from build123d import *

# Parameters (mm, degrees)
BOSS_EXTRUDE1_DEPTH = 2.032
FILLET1_R           = 2
SKETCH4_R           = 1.2446
CUT_EXTRUDE1_DEPTH  = 75.115872934
CUT_EXTRUDE2_DEPTH  = 75.115872934


with BuildPart() as part:
    # Sketch3 → Boss-Extrude1 (new body)
    with BuildSketch(Plane.XY):
        with BuildLine():
            Line((62.980794963, 30.66873734), (50.569205037, 30.66873734))
            ThreePointArc((50.569205037, 30.66873734), (45.275, 28.075), (39.980794963, 30.66873734))
            Line((39.980794963, 30.66873734), (27.569205037, 30.66873734))
            ThreePointArc((27.569205037, 30.66873734), (22.275, 28.075), (16.980794963, 30.66873734))
            Line((16.980794963, 30.66873734), (10.658308864, 17.473983742))
            ThreePointArc((10.658308864, 17.473983742), (13.670205209, 16.817167392), (16.069205037, 14.88126266))
            Line((16.069205037, 14.88126266), (28.480794963, 14.88126266))
            ThreePointArc((28.480794963, 14.88126266), (33.775, 17.475), (39.069205037, 14.88126266))
            Line((39.069205037, 14.88126266), (51.480794963, 14.88126266))
            ThreePointArc((51.480794963, 14.88126266), (56.775, 17.475), (62.069205037, 14.88126266))
            Line((62.069205037, 14.88126266), (68.391691136, 28.076016258))
            ThreePointArc((68.391691136, 28.076016258), (65.379794791, 28.732832608), (62.980794963, 30.66873734))
        make_face()
    extrude(amount=BOSS_EXTRUDE1_DEPTH)

    # Fillet1
    fillet1_edges = [part.edges().sort_by_distance(p)[0] for p in [
        (68.391691136, 28.076016258, 1.016),
        (62.069205037, 14.88126266, 1.016),
        (51.480794963, 14.88126266, 1.016),
        (39.069205037, 14.88126266, 1.016),
        (28.480794963, 14.88126266, 1.016),
        (16.069205037, 14.88126266, 1.016),
        (10.658308864, 17.473983742, 1.016),
        (16.980794963, 30.66873734, 1.016),
        (27.569205037, 30.66873734, 1.016),
        (39.980794963, 30.66873734, 1.016),
        (50.569205037, 30.66873734, 1.016),
        (62.980794963, 30.66873734, 1.016),
    ]]
    fillet(fillet1_edges, radius=FILLET1_R)

    # Sketch4 → Cut-Extrude1 (cut, through all)
    with BuildSketch(Plane.XY.offset(2.032)):
        with Locations((22.275, 20.49206771)):
            Circle(SKETCH4_R)
        with Locations((56.775, 25.307013878)):
            Circle(SKETCH4_R)
    extrude(amount=-CUT_EXTRUDE1_DEPTH, mode=Mode.SUBTRACT)

    # Sketch6 → Cut-Extrude2 (cut, through all)
    with BuildSketch(Plane.XY.offset(2.032)):
        with BuildLine():
            Line((62.077939702, 30.66873734), (51.472060298, 30.66873734))
            ThreePointArc((51.472060298, 30.66873734), (50.699880618, 30.513659708), (50.047448735, 30.072475883))
            ThreePointArc((50.047448735, 30.072475883), (45.275, 28.075), (40.502551265, 30.072475883))
            ThreePointArc((40.502551265, 30.072475883), (39.850119382, 30.513659708), (39.077939702, 30.66873734))
            Line((39.077939702, 30.66873734), (28.472060298, 30.66873734))
            ThreePointArc((28.472060298, 30.66873734), (27.699880618, 30.513659708), (27.047448735, 30.072475883))
            ThreePointArc((27.047448735, 30.072475883), (23.046259875, 28.119539219), (18.704481797, 29.105661435))
            ThreePointArc((18.704481797, 29.105661435), (17.084104729, 29.334902549), (15.835023411, 28.277561926))
            Line((15.835023411, 28.277561926), (11.804080417, 19.865159157))
            ThreePointArc((11.804080417, 19.865159157), (11.762608918, 18.229172162), (12.956514205, 17.109902981))
            ThreePointArc((12.956514205, 17.109902981), (14.346493431, 16.443724254), (15.547448735, 15.477524117))
            ThreePointArc((15.547448735, 15.477524117), (16.199880618, 15.036340292), (16.972060298, 14.88126266))
            Line((16.972060298, 14.88126266), (27.577939702, 14.88126266))
            ThreePointArc((27.577939702, 14.88126266), (28.350119382, 15.036340292), (29.002551265, 15.477524117))
            ThreePointArc((29.002551265, 15.477524117), (33.775, 17.475), (38.547448735, 15.477524117))
            ThreePointArc((38.547448735, 15.477524117), (39.199880618, 15.036340292), (39.972060298, 14.88126266))
            Line((39.972060298, 14.88126266), (50.577939702, 14.88126266))
            ThreePointArc((50.577939702, 14.88126266), (51.350119382, 15.036340292), (52.002551265, 15.477524117))
            ThreePointArc((52.002551265, 15.477524117), (56.003740125, 17.430460781), (60.345518203, 16.444338565))
            ThreePointArc((60.345518203, 16.444338565), (61.965895271, 16.215097451), (63.214976589, 17.272438074))
            Line((63.214976589, 17.272438074), (67.245919583, 25.684840843))
            ThreePointArc((67.245919583, 25.684840843), (67.287391082, 27.320827838), (66.093485795, 28.440097019))
            ThreePointArc((66.093485795, 28.440097019), (64.703506569, 29.106275746), (63.502551265, 30.072475883))
            ThreePointArc((63.502551265, 30.072475883), (62.850119382, 30.513659708), (62.077939702, 30.66873734))
        make_face()
        with BuildLine():
            Line((16.064084682, 28.1678034), (12.033141688, 19.755400631))
            ThreePointArc((12.033141688, 19.755400631), (11.99693707, 18.327183984), (13.039216385, 17.350061989))
            ThreePointArc((13.039216385, 17.350061989), (14.481890346, 16.658628129), (15.728374403, 15.655798912))
            ThreePointArc((15.728374403, 15.655798912), (16.297947437, 15.270645433), (16.972060298, 15.13526266))
            Line((16.972060298, 15.13526266), (27.577939702, 15.13526266))
            ThreePointArc((27.577939702, 15.13526266), (28.252052563, 15.270645433), (28.821625597, 15.655798912))
            ThreePointArc((28.821625597, 15.655798912), (33.775, 17.729), (38.728374403, 15.655798912))
            ThreePointArc((38.728374403, 15.655798912), (39.297947437, 15.270645433), (39.972060298, 15.13526266))
            Line((39.972060298, 15.13526266), (50.577939702, 15.13526266))
            ThreePointArc((50.577939702, 15.13526266), (51.252052563, 15.270645433), (51.821625597, 15.655798912))
            ThreePointArc((51.821625597, 15.655798912), (55.974501318, 17.682772279), (60.480878147, 16.659265728))
            ThreePointArc((60.480878147, 16.659265728), (61.895467327, 16.459138236), (62.985915318, 17.3821966))
            Line((62.985915318, 17.3821966), (67.016858312, 25.794599369))
            ThreePointArc((67.016858312, 25.794599369), (67.05306293, 27.222816016), (66.010783615, 28.199938011))
            ThreePointArc((66.010783615, 28.199938011), (64.568109654, 28.891371871), (63.321625597, 29.894201088))
            ThreePointArc((63.321625597, 29.894201088), (62.752052563, 30.279354567), (62.077939702, 30.41473734))
            Line((62.077939702, 30.41473734), (51.472060298, 30.41473734))
            ThreePointArc((51.472060298, 30.41473734), (50.797947437, 30.279354567), (50.228374403, 29.894201088))
            ThreePointArc((50.228374403, 29.894201088), (45.275, 27.821), (40.321625597, 29.894201088))
            ThreePointArc((40.321625597, 29.894201088), (39.752052563, 30.279354567), (39.077939702, 30.41473734))
            Line((39.077939702, 30.41473734), (28.472060298, 30.41473734))
            ThreePointArc((28.472060298, 30.41473734), (27.797947437, 30.279354567), (27.228374403, 29.894201088))
            ThreePointArc((27.228374403, 29.894201088), (23.075498682, 27.867227721), (18.569121853, 28.890734272))
            ThreePointArc((18.569121853, 28.890734272), (17.154532673, 29.090861764), (16.064084682, 28.1678034))
        make_face(mode=Mode.SUBTRACT)
    extrude(amount=-CUT_EXTRUDE2_DEPTH, mode=Mode.SUBTRACT)


solid = part.part
Could you check a few things on this model? Use its own coordinates, in mm. A direction names the side the tool comes from. Coordinates: 2 decimals unless noted, no trailing zeros. Write each loop counter-clockwise with the first axis right and the second up, starting at its lowest first coordinate (ties: lowest second). Pieces come first, ordered by that corner, then holes. Notation, with made-up numbers: (-27, -22) - (-20, -22) arc R13 ccw to (-20, -16) - close; hole circle Ø1 at (79.5, 1.5). An arc over 180 degrees is marked (long way). Write item = value, one per line.
1) Please list where these lines run through material, in increasing order: line 1 (X direction, y = 17, z = 0.2); line 2 (X direction, y = 19.75, z = 1.15); line 3 (X direction, y = 25.5, z = 0.6). Write a range as [from, to].
Result set:
line_1 = [13.87, 30.68], [36.87, 53.68], [59.87, 62.74]
line_2 = [12.03, 21.28], [23.27, 64.12]
line_3 = [14.79, 55.55], [58, 66.88]
2) Suppose I cut it at C-C on y = 18.25. Please give me the cut outline in (x, z).
Result set:
outline = (12.03, 0) - (63.4, 0) - (63.4, 2.03) - (12.03, 2.03) - close
3) Suppose I cut it at B-B on x = 31.5. Please give me the cut outline in (y, z).
Result set:
outline = (17.35, 0) - (30.41, 0) - (30.41, 2.03) - (17.35, 2.03) - close
4) We'd pull the mould along X, two halves only. Please class faces 1 (the cylindrical face through (14.463, 16.671, 1.03)), 2 (the cylindrical face through (23.141, 27.875, 1.03)), 3 (the flat face through (39, 23, 2.032)), 4 (the cylindrical face through (39.289, 15.274, 1.03)): +X half, -X half, draft (parallel to the pull), parting line (faces both ways), or undercut.
Result set:
face_1 = -X half
face_2 = undercut
face_3 = draft
face_4 = undercut
5) For faces 5 (the cylindrical face through (39.761, 30.276, 1.03)), 6 (the flat face through (34, 30.415, 1)), 7 (the cylindrical face through (28.243, 15.267, 1.03)), which set-ups out of +Z, -Z, +X, -X, +Y, -Y let a thin tool reach every point of the face, with its end or its side?
Result set:
face_5 = +Z, -Z, +Y
face_6 = +Z, -Z, +X, -X, +Y
face_7 = +Z, -Z, -Y
6) Suppose I cut it at A-A on z = 1.5. Please give me the cut outline in (x, y) (3 decimals).
Result set:
outline = (12.033, 19.755) arc R1.746 ccw to (13.039, 17.35) arc R6.954 cw to (15.728, 15.656) arc R1.746 ccw to (16.972, 15.135) - (27.578, 15.135) arc R1.746 ccw to (28.822, 15.656) arc R6.954 cw to (38.728, 15.656) arc R1.746 ccw to (39.972, 15.135) - (50.578, 15.135) arc R1.746 ccw to (51.822, 15.656) arc R6.954 cw to (60.481, 16.659) arc R1.746 ccw to (62.986, 17.382) - (67.017, 25.795) arc R1.746 ccw to (66.011, 28.2) arc R6.954 cw to (63.322, 29.894) arc R1.746 ccw to (62.078, 30.415) - (51.472, 30.415) arc R1.746 ccw to (50.228, 29.894) arc R6.954 cw to (40.322, 29.894) arc R1.746 ccw to (39.078, 30.415) - (28.472, 30.415) arc R1.746 ccw to (27.228, 29.894) arc R6.954 cw to (18.569, 28.891) arc R1.746 ccw to (16.064, 28.168) - close; hole circle Ø2.489 at (22.275, 20.492); hole circle Ø2.489 at (56.775, 25.307)
